Source: CAD feature listing. Evaluate the final solid. Frame: model axes, mm. Face numbers are marked on the shaded views. A direction names the side the tool comes from. Give positions to 0.01 mm unless a question says otherwise; leave off trailing zeros. Order: outer loops, then holes, each group sorted by start corner. A loop starts at its lowest first (then second) coordinate and runs counter-clockwise, first axis right, second up. Notation, with made-up numbers: M -37,-17.75 L -17,-17.75 A7 cw -17,-8.75 Z; hole C 78.5,62 d8. An arc over 180 degrees is marked long. Answer in a Markdown table with one row per item. Add a question column.
(1) Pin query (flat end, axial travel): P1, Ø1.5, axis at x = 13, y = 2, coming from the +Z side; P2, Ø0.6, axis at y = 3, z = 0, coming from the -X side; P3, Ø0.6, axis at x = 1, y = -3, coming from the -Z side. Return the tip coordinate at first contact, or that it passes through.
(2) Set-up query: the marked faces 1 and 2. Return all of +Z, -Z, +X, -X, +Y, -Y with unobstructed straight access to the full face (end or side cutting, diameter ignored); none if empty.
(3) Material intervals for line 1 along Z through (x, y) = (11, 0); line 2 along Y through (x, z) = (12, -1); line 3 along Z through (x, y) = (10, -1.75), sorted ascending.
(4) Section query A-A, the plane y = 0. Return loops of the section in (x, z), plus the area to 3 significant figures.
(5) Section query D-D, the plane y = -2.75. Return loops of the section in (x, z), plus the area to 3 significant figures.
(6) Section query C-C, the plane x = 9.5. Return loops of the section in (y, z).
(7) Mould query, pull axis Z, two halves, no side actions, for the marked faces 3, 4 and 5. Classes: pulls with the +Z half, pulls with the -Z half, needs draft (parallel to the pull), parting line crosses it, or undercut.
(8) Section query B-B, the plane z = 0. Return loops of the section in (x, y), plus the area to 3 significant figures.
Autodesk Inventor part; units mm, degrees
ref_plane "Work Plane1" through (0, 4, 0) normal (0, 1, 0) x (-1, 0, 0)
ref_plane "YZ Plane" through (0, 0, 0) normal (1, 0, 0) x (0, 1, 0)
ref_plane "XY Plane" through (0, 0, 0) normal (0, 0, 1) x (1, 0, 0)
sketch "Sketch1" plane through (0, 0, 0) normal (1, 0, 0) x (0, 1, 0)
  circle A0 centre (0, 0) radius 4
  circle A1 centre (0, 0) radius 2
  dimension "d0" = 8
  dimension "d1" = 4
extrude "Extrusion1" add sketch "Sketch1" along normal blind 18
ref_plane "Work Plane1" through (0, 4, 0) normal (0, 1, 0) x (-1, 0, 0)
sketch "Sketch2" plane through (0, 4, 0) normal (0, 1, 0) x (-1, 0, 0)
  line L0 (-18, 4) -> (-18, -4)
  line L1 (0, 4) -> (0, -4)
  line L2 (1, 1) -> (-3, 1)
  line L3 (-3, 1) -> (-3, -1)
  line L4 (-3, -1) -> (1, -1)
  line L5 (1, -1) -> (1, 1)
  point P0 (0, 0)
  point P1 (-1, -1)
  point P2 (0, 0)
  dimension "d4" = 1
  dimension "d5" = 1
  dimension "d6" = 3
extrude "Extrusion2" cut sketch "Sketch2" against normal through all
thread "Thread1"
properties part number "HUDSON-1-89B"
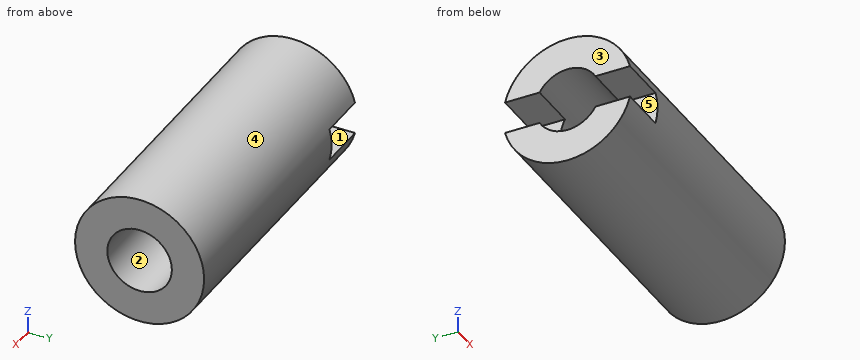
Values follow:
| question | item | result |
|---|---|---|
| 1 | P1 | stops at z = 3.8 |
| 1 | P2 | stops at x = 3 |
| 1 | P3 | stops at z = -2.95 |
| 2 | face 1 | -X, +Y, -Y |
| 2 | face 2 | +X, -X |
| 3 | line 1 | z = -4 to -2, 2 to 4 |
| 3 | line 2 | y = -3.87 to -1.73, 1.73 to 3.87 |
| 3 | line 3 | z = -3.6 to -0.97, 0.97 to 3.6 |
| 4 | outline | M 0,-4 L 18,-4 L 18,-2 L 0,-2 Z; M 0,2 L 18,2 L 18,4 L 0,4 Z |
| 4 | area | 72.0 mm² |
| 5 | outline | M 0,-2.9 L 18,-2.9 L 18,2.9 L 0,2.9 L 0,1 L 3,1 L 3,-1 L 0,-1 Z |
| 5 | area | 98.6 mm² |
| 6 | outline | C 0,0 d8; hole C 0,0 d4 |
| 7 | face 3 | needs draft |
| 7 | face 4 | parting line crosses it |
| 7 | face 5 | undercut |
| 8 | outline | M 3,-4 L 18,-4 L 18,-2 L 3,-2 Z; M 3,2 L 18,2 L 18,4 L 3,4 Z |
| 8 | area | 60.0 mm² |
